Drawing for the job (mm, zero at the part's lowest x, y, z). A direction names the side the tool comes from. Round coordinates to 2 decimals unless told otherwise and drop trailing zeros. Write each loop counter-clockwise with the first axis right and the second up, starting at its lowest first coordinate (ties: lowest second). Pieces come first, ordered by that corner, then holes. Notation, with made-up numbers: (-17, 60) -> (4, 60) arc R30 ccw to (4, 93) -> close; hole circle Ø10 at (69, 70). An arc over 180 degrees is marked (long way). Answer in a Markdown table with one row per item. Add a question column.
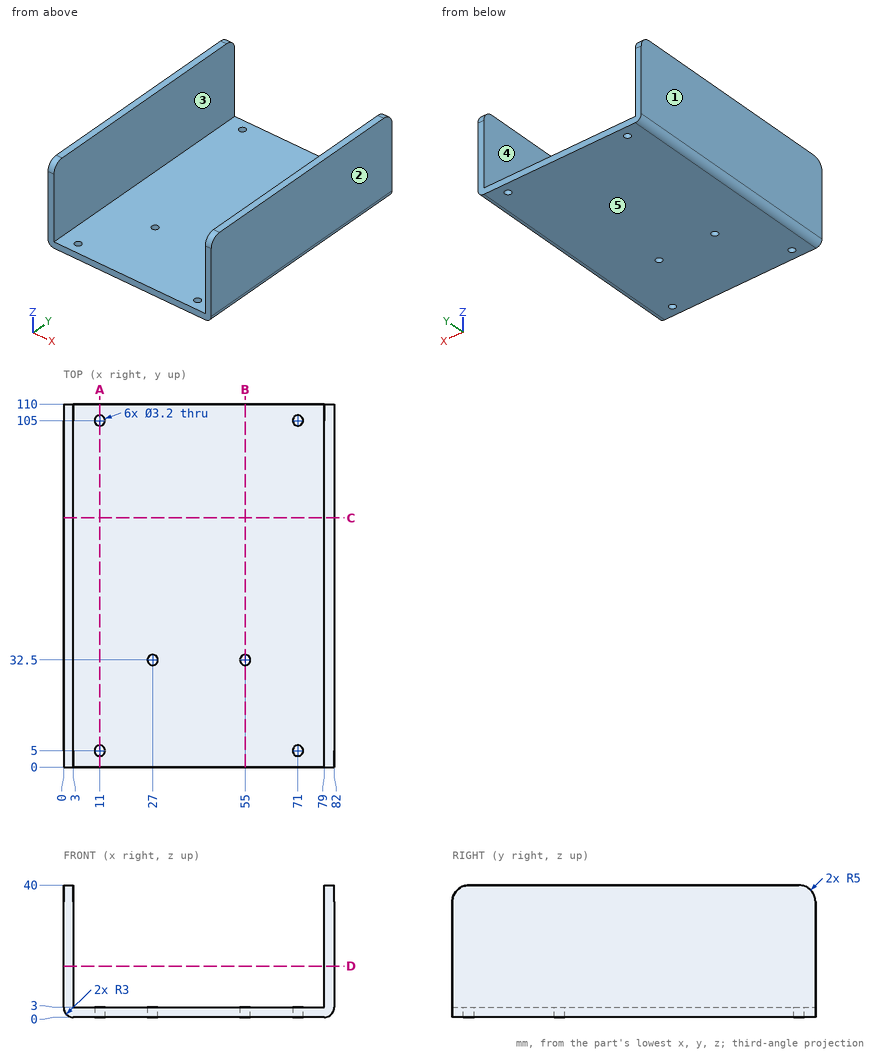
(1) Saw through at A-A (x = 11). List the corners of the cut face in (y, z), plus the area to 3 significant figures.
(2) Drop flat-ended pins along their axis: P1, Ø2.5, axis at x = 27, y = 32.5, coming from the -Z side; P2, Ø3, axis at x = 56.5, y = 50, coming from the +Z side. Give the stop position or say it passes through.
(3) Saw through at D-D (z = 15.5). List the corners of the cut face in (x, y).
(4) Which spindle directions (+Z, -Z, +X, -X, +Y, -Y) get a long thin tool onto all of the face, cutting with end or side? Do the marked faces 4 and 5. Say none if no direction does.
(5) Saw through at B-B (x = 55). List the corners of the cut face in (y, z), plus the area to 3 significant figures.
(6) Saw through at C-C (y = 75.5). List the corners of the cut face in (x, z), plus the area to 3 significant figures.
(7) Mould opens along X. For the marked faces 1, 2 and 3 say: pulls with the +X half, pulls with the -X half, needs draft (parallel to the pull), parting line crosses it, or undercut.
(8) Probe line 1 along Y through (x, z) = (71, 2.25); line 2 along Y through (x, z) = (55, 1.7); line 3 along X through (y, z) = (39, 33.5). List the from-to ranges inside material, lowest first.
Answer sheet:
| question | item | result |
|---|---|---|
| 1 | outline | (0, 0) -> (3.4, 0) -> (3.4, 3) -> (0, 3) -> close; (6.6, 0) -> (103.4, 0) -> (103.4, 3) -> (6.6, 3) -> close; (106.6, 0) -> (110, 0) -> (110, 3) -> (106.6, 3) -> close |
| 1 | area | 311 mm² |
| 2 | P1 | passes through |
| 2 | P2 | stops at z = 3 |
| 3 | outline | (0, 0) -> (3, 0) -> (3, 110) -> (0, 110) -> close; (79, 0) -> (82, 0) -> (82, 110) -> (79, 110) -> close |
| 4 | face 4 | +Z, +Y, -Y |
| 4 | face 5 | -Z, +X, -X, +Y, -Y |
| 5 | outline | (0, 0) -> (30.9, 0) -> (30.9, 3) -> (0, 3) -> close; (34.1, 0) -> (110, 0) -> (110, 3) -> (34.1, 3) -> close |
| 5 | area | 320 mm² |
| 6 | outline | (0, 3) arc R3 ccw to (3, 0) -> (79, 0) arc R3 ccw to (82, 3) -> (82, 40) -> (79, 40) -> (79, 3) -> (3, 3) -> (3, 40) -> (0, 40) -> close |
| 6 | area | 464 mm² |
| 7 | face 1 | pulls with the -X half |
| 7 | face 2 | pulls with the +X half |
| 7 | face 3 | undercut |
| 8 | line 1 | y = 0 to 3.4, 6.6 to 103.4, 106.6 to 110 |
| 8 | line 2 | y = 0 to 30.9, 34.1 to 110 |
| 8 | line 3 | x = 0 to 3, 79 to 82 |
